Can you work these out from the model? Positions are in its coordinate system, mm. A direction names the side the tool comes from. Give positions to 0.01 mm unless a question says otherwise; leave off trailing zeros. Order: outer loops, then holes, each group sorted by start corner. A loop starts at its lowest first (then second) coordinate and runs counter-clockwise, first axis right, second up. Notation, with made-up numbers: (-26.5, 28) - (11.5, 28) arc R7 ccw to (11.5, 41) - close; hole circle Ø3 at (31, 32). An arc over 180 degrees is marked (long way). Answer as CSV lines item,"result".
```python
from build123d import *

# Parameters (mm, degrees)
SKETCH1_W           = 50.8
SKETCH1_H           = 55
SKETCH1_R           = 2.286
BOSS_EXTRUDE1_DEPTH = 8.89
FILLET1_R           = 7.62
SKETCH2_W           = 50.8
SKETCH2_H           = 25.4
BOSS_EXTRUDE2_DEPTH = 34.81959
FILLET2_R           = 7.62
SKETCH3_R           = 3.175
CUT_EXTRUDE1_DEPTH  = 41.2
LPATTERN1_COUNT     = 2
LPATTERN1_PITCH     = 16.51


with BuildPart() as part:
    # Sketch1 → Boss-Extrude1 (new body)
    with BuildSketch(Plane(origin=(0, 0, 0), x_dir=(0, 0, -1), z_dir=(1, 0, 0))):
        Rectangle(SKETCH1_W, SKETCH1_H)
        with Locations((-10, 20)):
            Circle(SKETCH1_R, mode=Mode.SUBTRACT)
        with Locations((10, 20)):
            Circle(SKETCH1_R, mode=Mode.SUBTRACT)
        with Locations((-10, -20)):
            Circle(SKETCH1_R, mode=Mode.SUBTRACT)
        with Locations((10, -20)):
            Circle(SKETCH1_R, mode=Mode.SUBTRACT)
    extrude(amount=BOSS_EXTRUDE1_DEPTH)

    # Fillet1
    fillet1_edges = [part.edges().sort_by_distance(p)[0] for p in [
        (4.445, 27.5, 25.4),
        (4.445, 27.5, -25.4),
        (4.445, -27.5, -25.4),
        (4.445, -27.5, 25.4),
    ]]
    fillet(fillet1_edges, radius=FILLET1_R)

    # Sketch2 → Boss-Extrude2 (add)
    with BuildSketch(Plane(origin=(8.89, 0, 0), x_dir=(0, 0, -1), z_dir=(1, 0, 0))):
        Rectangle(SKETCH2_W, SKETCH2_H)
    extrude(amount=BOSS_EXTRUDE2_DEPTH)

    # Fillet2
    fillet2_edges = [part.edges().sort_by_distance(p)[0] for p in [
        (26.299795, 12.7, 25.4),
        (26.299795, -12.7, 25.4),
        (26.299795, -12.7, -25.4),
        (26.299795, 12.7, -25.4),
    ]]
    fillet(fillet2_edges, radius=FILLET2_R)

    # Mirror6: part across plane


with BuildPart() as part_1:
    add(part.part)
    add(part.part.mirror(Plane(origin=(43.70959, 0, 0), x_dir=(0, 0, 1), z_dir=(1, 0, 0))))

    # Sketch3 → Cut-Extrude1 (cut, through all)
    with BuildSketch(Plane(origin=(0, 12.7, 0), x_dir=(1, 0, 0), z_dir=(0, 1, 0))):
        with Locations((53.23459, 8.255)):
            Circle(SKETCH3_R)
        with Locations((34.18459, 8.255)):
            Circle(SKETCH3_R)
    cut_extrude1 = extrude(amount=-CUT_EXTRUDE1_DEPTH, mode=Mode.SUBTRACT)

    # LPattern1: Cut-Extrude1 ×2
    with Locations(*[(0, 0, i * LPATTERN1_PITCH) for i in range(1, LPATTERN1_COUNT)]):
        add(cut_extrude1, mode=Mode.SUBTRACT)


solid = part_1.part
```
1) I want a section at D-D on z = -10. Count the separate pieces of the cut face and the enclosed holes in it, plus the area to 3 significant figures.
Answer block:
separate pieces,"7"
enclosed holes,"0"
area,"2,310 mm2"
2) I want a section at A-A on x = 25. Write out the boundary of the cut face in (y, z).
Answer block:
outline,"(-12.7, -17.78) arc R7.62 ccw to (-5.08, -25.4) - (5.08, -25.4) arc R7.62 ccw to (12.7, -17.78) - (12.7, 17.78) arc R7.62 ccw to (5.08, 25.4) - (-5.08, 25.4) arc R7.62 ccw to (-12.7, 17.78) - close"
3) I'm going to push flat-ended pins straight in: P1, Ø3, axis at x = 50, z = 6, coming from the -Y side; P2, Ø3, axis at x = 51.5, z = 9.5, coming from the +Y side. Where does each tip first touch, or does it pass through?
Answer block:
P1,"y = -12.7"
P2,"y = 12.7"
4) I want a section at C-C on z = 14. Write out the boundary of the cut face in (x, y).
Answer block:
outline,"(0, -27.5) - (8.89, -27.5) - (8.89, -12.7) - (78.53, -12.7) - (78.53, -27.5) - (87.42, -27.5) - (87.42, 27.5) - (78.53, 27.5) - (78.53, 12.7) - (8.89, 12.7) - (8.89, 27.5) - (0, 27.5) - close"
5) I need wall thicknesses on line 1 along Y through (x, z) = (82, 10); line 2 along X through (y, z) = (-19.5, -4); line 3 along X through (y, z) = (10, -10). Which ranges of each line are inside material? Lowest first, please. Write a range as [from, to].
Answer block:
line 1,"[-27.5, -22.29], [-17.71, 17.71], [22.29, 27.5]"
line 2,"[0, 8.89], [78.53, 87.42]"
line 3,"[0, 31.53], [36.84, 50.58], [55.89, 87.42]"
6) Which directions (+Z, -Z, +X, -X, +Y, -Y) give clear straight access to the entire face, cutting with the end or side of a thin tool? Please do faces 1 (the cylindrical face through (43.222, -10.409, -23.227)), 2 (the cylindrical face through (4.507, 25.327, -23.109)), 3 (the cylindrical face through (43.222, 10.409, -23.227)).
Answer block:
face 1,"-Z, -Y"
face 2,"-Z, +X, -X, +Y"
face 3,"-Z, +Y"
7) If we mould it in two halves opening along Y, with no side actions, what happens to faces 4 (the flat face through (87.419, 0, 0)), 5 (the flat face through (44, -12.7, 0)), 6 (the cylindrical face through (83.04, 17.77, -9.5)), 7 (the cylindrical face through (4.507, 25.209, 23.227))? For each: +Y half, -Y half, draft (parallel to the pull), parting line (faces both ways), or undercut.
Answer block:
face 4,"draft"
face 5,"-Y half"
face 6,"undercut"
face 7,"+Y half"
8) I want a section at B-B on y = -3.5. Write out the boundary of the cut face in (x, z) (3 decimals), plus the area to 3 significant figures.
Answer block:
outline,"(0, -25.4) - (87.419, -25.4) - (87.419, 25.4) - (0, 25.4) - close; hole circle Ø6.35 at (34.185, -8.255); hole circle Ø6.35 at (34.185, 8.255); hole circle Ø6.35 at (53.235, -8.255); hole circle Ø6.35 at (53.235, 8.255)"
area,"4,310 mm2"
